Work out the finished part from the listing and answer in its coordinate system (mm). Face numbers are marked on the shaded views. Coordinates: 2 decimals unless noted, no trailing zeros. Write each loop counter-clockwise with the first axis right and the second up, starting at its lowest first coordinate (ties: lowest second). Pieces come first, ordered by that corner, then holes. Notation, with made-up numbers: (-9.75, 73.5) - (28.25, 73.5) arc R24 ccw to (28.25, 105.5) - close; hole circle Ø10 at (23.5, 61). An arc over 180 degrees is marked (long way). Use CSV: the item, a comma, the result in double quotes. Start each with the question number.
from build123d import *

# Parameters (mm, degrees)
SKETCH1_R           = 1.55
SKETCH1_R_2         = 1.3
SKETCH1_R_3         = 1.05
BOSS_EXTRUDE1_DEPTH = 4.5


with BuildPart() as part:
    # Sketch1 → Boss-Extrude1 (new body)
    with BuildSketch(Plane(origin=(0, 0, 0), x_dir=(1, 0, 0), z_dir=(0, 1, 0))):
        with BuildLine():
            Line((-26, -46), (26, -46))
            ThreePointArc((26, -46), (27.414213562, -45.414213562), (28, -44))
            Line((28, -44), (28, 44))
            ThreePointArc((28, 44), (27.414213562, 45.414213562), (26, 46))
            Line((26, 46), (-26, 46))
            ThreePointArc((-26, 46), (-27.414213562, 45.414213562), (-28, 44))
            Line((-28, 44), (-28, -44))
            ThreePointArc((-28, -44), (-27.414213562, -45.414213562), (-26, -46))
        make_face()
        with Locations(Location((24, 42, 0), (0, 0, 270))):
            Circle(SKETCH1_R, mode=Mode.SUBTRACT)
        with Locations(Location((24, -42, 0), (0, 0, 90))):
            Circle(SKETCH1_R, mode=Mode.SUBTRACT)
        with Locations(Location((-24, 42, 0), (0, 0, 90))):
            Circle(SKETCH1_R, mode=Mode.SUBTRACT)
        with Locations(Location((-24, -42, 0), (0, 0, 270))):
            Circle(SKETCH1_R, mode=Mode.SUBTRACT)
        with Locations(Location((-21.5, 21.5, 0), (0, 0, 270))):
            Circle(SKETCH1_R_2, mode=Mode.SUBTRACT)
        with Locations(Location((21.5, 21.5, 0), (0, 0, 90))):
            Circle(SKETCH1_R_2, mode=Mode.SUBTRACT)
        with Locations(Location((21.5, -21.5, 0), (0, 0, 270))):
            Circle(SKETCH1_R_2, mode=Mode.SUBTRACT)
        with Locations(Location((-21.5, -21.5, 0), (0, 0, 90))):
            Circle(SKETCH1_R_2, mode=Mode.SUBTRACT)
        with Locations(Location((0, 25, 0), (0, 0, 270))):
            Circle(SKETCH1_R_3, mode=Mode.SUBTRACT)
        with Locations(Location((0, -25, 0), (0, 0, 90))):
            Circle(SKETCH1_R_3, mode=Mode.SUBTRACT)
    extrude(amount=BOSS_EXTRUDE1_DEPTH)


solid = part.part
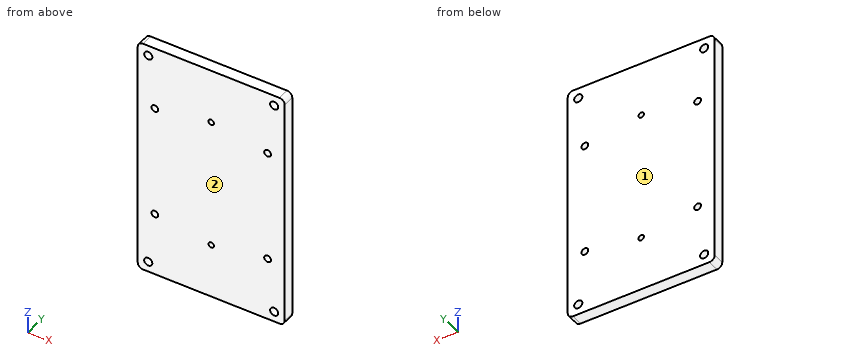
Item 1: Straight lines are drawn through the part: probe 1 along X at (y, z) = (2.8, 42); probe 2 along X at (y, z) = (1.5, -21.5); probe 3 along Z at (x, y) = (-21, 2.15). For each, find the intervals that lie inside material, in ascending order. Write a range as [from, to].
Item 2: A cutting plane is placed at C-C (x = 0). Determine the outline of the cut face in (y, z).
Item 3: Determine the mould class of the marked faces 1 and 2 for opening direction Y: +Y half, -Y half, draft (parallel to the pull), parting line (faces both ways), or undercut.
Item 4: A cutting plane is placed at A-A (x = 21.5). Determine the outline of the cut face in (y, z), then the cut area to 3 significant figures.
Item 5: A cutting plane is placed at B-B (z = 25). Determine the outline of the cut face in (x, y), then the cut area to 3 significant figures.
Calculated:
1,probe 1,"x = [-28, -25.55], [-22.45, 22.45], [25.55, 28]"
1,probe 2,"x = [-28, -22.8], [-20.2, 20.2], [22.8, 28]"
1,probe 3,"z = [-46, -22.7], [-20.3, 20.3], [22.7, 46]"
2,outline,"(0, -46) - (4.5, -46) - (4.5, -26.05) - (0, -26.05) - close; (0, -23.95) - (4.5, -23.95) - (4.5, 23.95) - (0, 23.95) - close; (0, 26.05) - (4.5, 26.05) - (4.5, 46) - (0, 46) - close"
3,face 1,"+Y half"
3,face 2,"-Y half"
4,outline,"(0, -46) - (4.5, -46) - (4.5, -22.8) - (0, -22.8) - close; (0, -20.2) - (4.5, -20.2) - (4.5, 20.2) - (0, 20.2) - close; (0, 22.8) - (4.5, 22.8) - (4.5, 46) - (0, 46) - close"
4,area,"391 mm²"
5,outline,"(-28, 0) - (-1.05, 0) - (-1.05, 4.5) - (-28, 4.5) - close; (1.05, 0) - (28, 0) - (28, 4.5) - (1.05, 4.5) - close"
5,area,"243 mm²"
